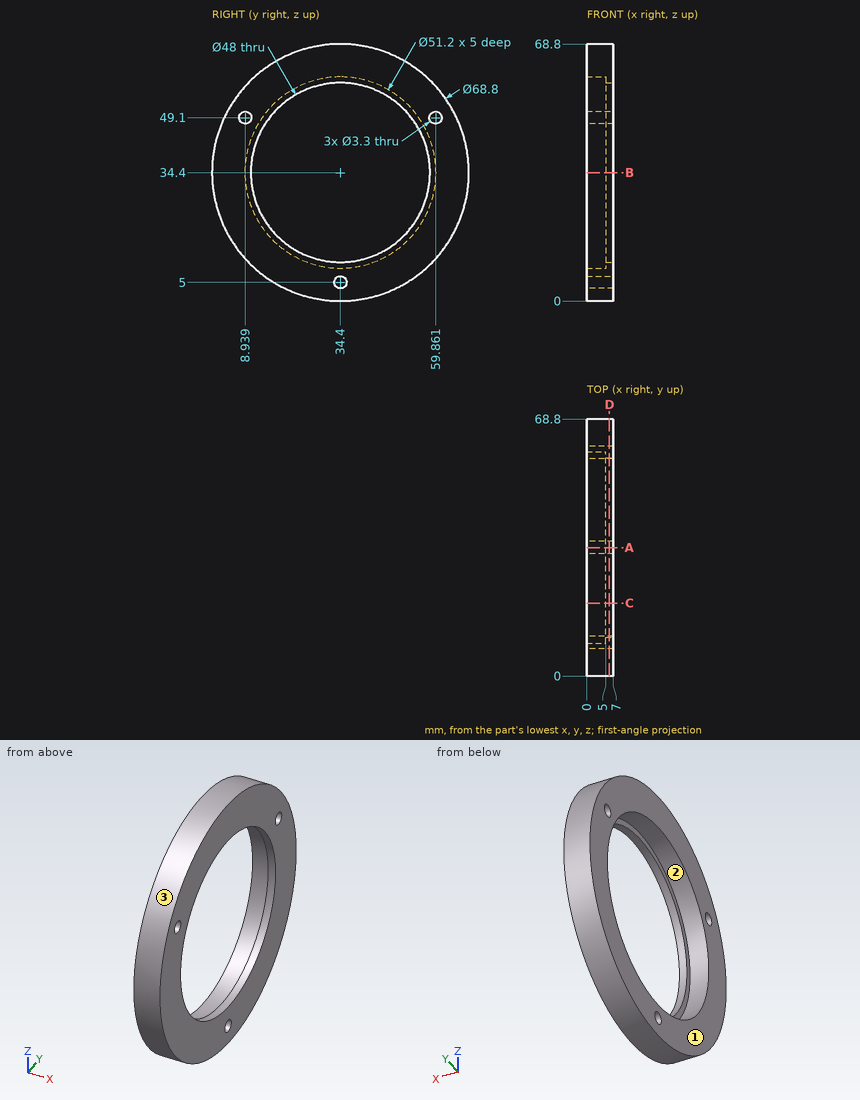
Geometry: see drawing. Coordinates: mm, zero at the bounding-box minimum. Round coordinates to 2 decimals unless told otherwise and drop trailing zeros. Write each loop counter-clockwise with the first axis right and the second up, starting at its lowest first coordinate (ties: lowest second). Pieces come first, ordered by that corner, then holes.
Item 1: Section query A-A (y = 34.4). Return loops of the section in (x, z).
Item 2: Pin query (flat end, axial travel): P1, Ø3, axis at x = 1.5, y = 27.5, coming from the +Z side; P2, Ø3, axis at x = 2.5, y = 10, coming from the +Z side; P3, Ø1, axis at x = 5, z = 8.5, coming from the +Y side. Return the tip coordinate at first contact, or that it passes through.
Item 3: Section query B-B (z = 34.4). Return loops of the section in (x, y).
Item 4: Section query C-C (y = 19.5). Return loops of the section in (x, z), plus the area to 3 significant figures.
Item 5: Section query D-D (x = 6). Return loops of the section in (y, z), plus the area to 3 significant figures.
Item 6: Mould query, pull axis Z, two halves, no side actions, for the marked faces 1, 2 and 3. Classes: +Z half, -Z half, draft (parallel to the pull), parting line (faces both ways), or undercut.
Item 7: Material intervals for L1, parallel to Y at x = 2.7, z = 34.4; L2, parallel to Y at x = 5.65, z = 34.4; L3, parallel to Y at x = 2.5, z = 49.1, sorted ascending.
Completed:
1. outline: (0, 0) - (7, 0) - (7, 3.35) - (0, 3.35) - close; (0, 6.65) - (7, 6.65) - (7, 10.4) - (5, 10.4) - (5, 8.8) - (0, 8.8) - close; (0, 60) - (5, 60) - (5, 58.4) - (7, 58.4) - (7, 68.8) - (0, 68.8) - close
2. P1: stops at z = 68.37
2. P2: stops at z = 60.07
2. P3: stops at y = 57.6
3. outline: (0, 0) - (7, 0) - (7, 10.4) - (5, 10.4) - (5, 8.8) - (0, 8.8) - close; (0, 60) - (5, 60) - (5, 58.4) - (7, 58.4) - (7, 68.8) - (0, 68.8) - close
4. outline: (0, 3.39) - (7, 3.39) - (7, 15.59) - (5, 15.59) - (5, 13.58) - (0, 13.58) - close; (0, 55.22) - (5, 55.22) - (5, 53.21) - (7, 53.21) - (7, 65.41) - (0, 65.41) - close
4. area: 151 mm2
5. outline: circle Ø68.8 at (34.4, 34.4); hole circle Ø3.3 at (8.94, 49.1); hole circle Ø48 at (34.4, 34.4); hole circle Ø3.3 at (34.4, 5); hole circle Ø3.3 at (59.86, 49.1)
5. area: 1,880 mm2
6. face 1: draft
6. face 2: undercut
6. face 3: parting line
7. L1: y = 0 to 8.8, 60 to 68.8
7. L2: y = 0 to 10.4, 58.4 to 68.8
7. L3: y = 3.3 to 7.29, 10.59 to 13.44, 55.36 to 58.21, 61.51 to 65.5
